Can you work these out from the model? Positions are in its coordinate system, mm. Face numbers are marked on the shaded views. A direction names the side the tool comes from. Coordinates: 2 decimals unless noted, no trailing zeros. Write each loop counter-clockwise with the first axis right and the second up, starting at its lowest first coordinate (ties: lowest second). Pieces come first, ordered by that corner, then holes.
```python
from build123d import *

# Parameters (mm, degrees)
BOSS_EXTRUDE1_DEPTH = 12.7
SKETCH2_R           = 2.675
CUT_EXTRUDE1_DEPTH  = 16.24
SKETCH3_W           = 7.62
SKETCH3_H           = 3.81
CUT_EXTRUDE2_DEPTH  = 104.7100001


with BuildPart() as part:
    # Sketch1 → Boss-Extrude1 (new body)
    with BuildSketch(Plane.XY):
        with BuildLine():
            Line((-51.855, 0), (51.855, 0))
            Line((51.855, 0), (51.855, -15.24))
            ThreePointArc((51.855, -15.24), (0, -9.602362237), (-51.855, -15.24))
            Line((-51.855, -15.24), (-51.855, 0))
        make_face()
    extrude(amount=BOSS_EXTRUDE1_DEPTH)

    # Sketch2 → Cut-Extrude1 (cut, through all)
    with BuildSketch(Plane(origin=(0, 0, 0), x_dir=(1, 0, 0), z_dir=(0, 1, 0))):
        with Locations((-44.855, -6.35)):
            Circle(SKETCH2_R)
        with Locations((44.855, -6.35)):
            Circle(SKETCH2_R)
    extrude(amount=-CUT_EXTRUDE1_DEPTH, mode=Mode.SUBTRACT)

    # Sketch3 → Cut-Extrude2 (cut, through all)
    with BuildSketch(Plane(origin=(51.855, 0, 0), x_dir=(0, 0, -1), z_dir=(1, 0, 0))):
        with Locations((-6.35, -13.335)):
            Rectangle(SKETCH3_W, SKETCH3_H)
    extrude(amount=-CUT_EXTRUDE2_DEPTH, mode=Mode.SUBTRACT)


solid = part.part
```
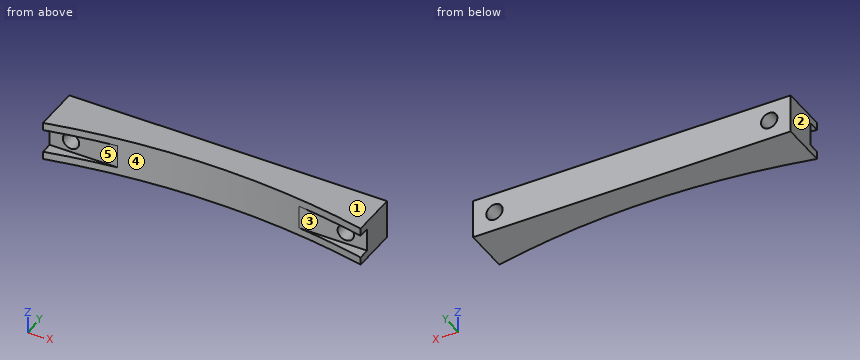
1. If I drill on L1, parallel to X at y = -6.25, z = 6.35 (3 decimals); L2, parallel to X at y = -1, z = 7.75 (3 decimals); L3, parallel to Y at x = 32, z = 9.5, over which ranges is the centre line in solid material (lowest first)?
2. If we section it at B-B, the plane y = -8.75: List the corners of the cut face in (x, z) for me (3 decimals).
3. If we section it at A-A, the plane z = 6.35: List the corners of the cut face in (x, y) for me (1 decimal).
4. Which directions (+Z, -Z, +X, -X, +Y, -Y) give clear straight access to the entire face, cutting with the end or side of a thin tool? Please do the marked faces 4 and 5.
5. If we section it at D-D, the plane z = 1.5: List the corners of the cut face in (x, y) for me (3 decimals), plus the area to 3 significant figures.
6. I'm going to push flat-ended pins straight in: P1, Ø2, axis at x = -9.5, z = 4, coming from the -Y side; P2, Ø6, axis at x = -44.855, z = 6.35, coming from the -Y side; P3, Ø1, axis at y = -12, z = 7.5, coming from the +X side; P4, Ø6, axis at x = -44.5, z = 7.5, coming from the -Y side. Where does each tip first touch, or does it pass through?
7. We'd pull the mould along Z, two halves only. Please class the marked faces 1, 2 and 3: released by +Z, released by -Z, zero draft, split by the parting line, or undercut.
Answers:
1. L1: x = -51.855 to -47.53, -42.18 to 42.18, 47.53 to 51.855
1. L2: x = -51.855 to -47.134, -42.576 to 42.576, 47.134 to 51.855
1. L3: y = -11.43 to 0
2. outline: (-51.855, 0) - (51.855, 0) - (51.855, 12.7) - (-51.855, 12.7) - close; hole circle Ø5.35 at (-44.855, 6.35); hole circle Ø5.35 at (44.855, 6.35)
3. outline: (-51.9, -11.4) - (-47.5, -11.4) - (-47.5, 0) - (-51.9, 0) - close; (-42.2, -11.4) - (-29.6, -11.4) arc R241.3 cw to (29.6, -11.4) - (42.2, -11.4) - (42.2, 0) - (-42.2, 0) - close; (47.5, -11.4) - (51.9, -11.4) - (51.9, 0) - (47.5, 0) - close
4. face 4: +Z, -Z, -Y
4. face 5: +X, -X, -Y
5. outline: (-51.855, -15.24) arc R241.3 cw to (51.855, -15.24) - (51.855, 0) - (-51.855, 0) - close
5. area: 1,190 mm2
6. P1: stops at y = -9.83
6. P2: stops at y = -11.43
6. P3: passes through
6. P4: stops at y = -14.01
7. face 1: released by +Z
7. face 2: zero draft
7. face 3: undercut
